Check sheet for the modelled part. Datum: model origin and axes. Units: mm. Face numbers are marked on the shaded views. A direction names the side the tool comes from. Give positions to 0.01 mm unless a question says otherwise; leave off trailing zeros. Loops run counter-clockwise (first coordinate to the right, second up) from the corner with the lowest first, then second, coordinate; pieces in that order, holes last. Notation, with made-up numbers: M 69,-4 L 101,-4 A22 cw 101,18 Z; hole C -20,28 d3. An arc over 180 degrees is marked long. Use one line per item in the form item = value.
from build123d import *

# Parameters (mm, degrees)
BOSS_EXTRU_1_DEPTH      = 6
ESQUISSE2_R             = 1.5
ENL_V_MAT_EXTRU_1_DEPTH = 94.914855055


with BuildPart() as part:
    # Esquisse1 → Boss.-Extru.1 (new body)
    with BuildSketch(Plane.XY):
        Polygon((0, 0), (-66, 0), (-66, 20), (-72, 20), (-72, 40), (-66, 40), (-66, 60), (0, 60), (0, 40), (-6, 40), (-6, 20), (0, 20), align=None)
    extrude(amount=BOSS_EXTRU_1_DEPTH)

    # Esquisse2 → Enlèv. mat.-Extru.1 (cut, through all)
    with BuildSketch(Plane(origin=(0, 0, 0), x_dir=(-1, 0, 0), z_dir=(0, 0, -1))):
        with Locations(Location((3, 50, 0), (0, 0, 180))):
            Circle(ESQUISSE2_R)
        with Locations((3, 10)):
            Circle(ESQUISSE2_R)
    extrude(amount=-ENL_V_MAT_EXTRU_1_DEPTH, mode=Mode.SUBTRACT)


solid = part.part
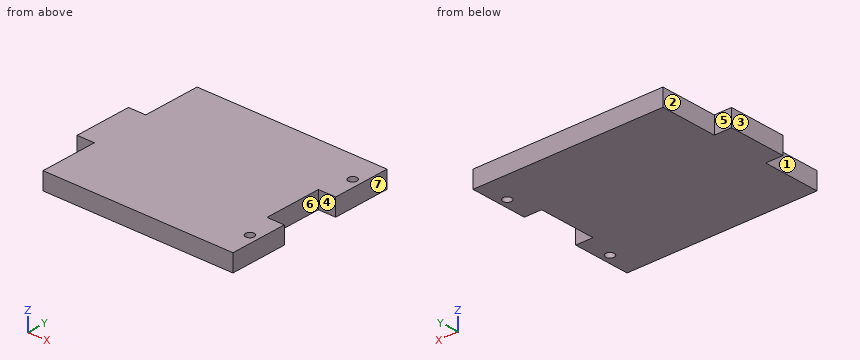
1) Section check C-C (z = 1.6). Record the cut outline in (x, y).
Evaluation:
outline = M -72,20 L -66,20 L -66,0 L 0,0 L 0,20 L -6,20 L -6,40 L 0,40 L 0,60 L -66,60 L -66,40 L -72,40 Z; hole C -3,10 d3; hole C -3,50 d3
2) Scan lines: line 1 (Y direction, x = -3, z = 1.7); line 2 (Y direction, x = -5.5, z = 3.75); line 3 (X direction, y = 50, z = 4.4). Record each from-to range of solid material in increasing order.
Evaluation:
line_1 = 0 to 8.5, 11.5 to 20, 40 to 48.5, 51.5 to 60
line_2 = 0 to 20, 40 to 60
line_3 = -66 to -4.5, -1.5 to 0
3) Release check for a two-part mould opening along Y. For the marked faces 4, 5, 6 and 7 record: pulls with the +Y half, pulls with the -Y half, needs draft (parallel to the pull), parting line crosses it, or undercut.
Evaluation:
face_4 = undercut
face_5 = pulls with the +Y half
face_6 = undercut
face_7 = needs draft
4) Section check D-D (y = 35.5). Record the cut outline in (x, z), then the cut area to 3 significant figures.
Evaluation:
outline = M -72,0 L -6,0 L -6,6 L -72,6 Z
area = 396 mm^2
5) Section check B-B (y = 50). Record the cut outline in (x, z).
Evaluation:
outline = M -66,0 L -4.5,0 L -4.5,6 L -66,6 Z; M -1.5,0 L 0,0 L 0,6 L -1.5,6 Z
6) Depth check by flat-ended pin: pin 1 Ø3 at (y, z) = (12.5, 3) entering from -X; pin 2 Ø2.5 at (x, y) = (-3, 50) entering from +Z (3 decimals); pin 3 Ø1.8 at (x, z) = (-70.5, 4) entering from -Y. Enter the tip coordinate at first touch or a pass-through.
Evaluation:
pin_1 = -66
pin_2 = through
pin_3 = 20
7) Section check A-A (x = -3). Record the cut outline in (y, z).
Evaluation:
outline = M 0,0 L 8.5,0 L 8.5,6 L 0,6 Z; M 11.5,0 L 20,0 L 20,6 L 11.5,6 Z; M 40,0 L 48.5,0 L 48.5,6 L 40,6 Z; M 51.5,0 L 60,0 L 60,6 L 51.5,6 Z
8) Set-up check for the marked faces 1, 2 and 3: record each of +Z, -Z, +X, -X, +Y, -Y from which the full face is reachable in a straight line by a thin tool's end or side.
Evaluation:
face_1 = +Z, -Z, -X, -Y
face_2 = +Z, -Z, -X, +Y
face_3 = +Z, -Z, -X, +Y, -Y
